from build123d import *

# Parameters (mm, degrees)
SKETCH1_R                    = 11.5
BOSS_EXTRUDE1_DEPTH          = 100
FILLET1_R                    = 8
SKETCH2_R                    = 4.1
SKETCH2_R_2                  = 6
CUT_EXTRUDE1_DEPTH           = 10
BOSS_EXTRUDE2_START          = 20
SKETCH3_R                    = 4.1
SKETCH3_R_2                  = 6
BOSS_EXTRUDE2_DEPTH          = 20
FILLET2_R                    = 3
CUT_EXTRUDE_THIN1_DEPTH      = 184.360351078
CUT_EXTRUDE_THIN1_DEPTH_BACK = 20
CUT_EXTRUDE_THIN2_DEPTH      = 164.298096582
CUT_EXTRUDE_THIN2_DEPTH_BACK = 20
FILLET3_R                    = 3
CUT_EXTRUDE2_DEPTH           = 161.944923335
CUT_EXTRUDE2_DEPTH_BACK      = 161.944923335
SKETCH6_R                    = 2.25
CUT_EXTRUDE3_DEPTH           = 3


with BuildPart() as part:
    # Sketch1 → Boss-Extrude1 (new body)
    with BuildSketch(Plane(origin=(0, 0, 0), x_dir=(1, 0, 0), z_dir=(0, 1, 0))):
        with BuildLine():
            Line((137.460581558, -14.5), (119.460581558, -14.5))
            Line((119.460581558, -14.5), (119.460581558, 11.5))
            Line((119.460581558, 11.5), (-24.539418442, 11.5))
            Line((-24.539418442, 11.5), (-24.539418442, -14.5))
            Line((-24.539418442, -14.5), (-42.539418442, -14.5))
            ThreePointArc((-42.539418442, -14.5), (-57.039418442, 0), (-42.539418442, 14.5))
            Line((-42.539418442, 14.5), (137.460581558, 14.5))
            ThreePointArc((137.460581558, 14.5), (151.960581558, 0), (137.460581558, -14.5))
        make_face()
        with Locations(Location((-42.539418442, 0, 0), (0, 0, 270))):
            Circle(SKETCH1_R, mode=Mode.SUBTRACT)
        with Locations(Location((137.460581558, 0, 0), (0, 0, 270))):
            Circle(SKETCH1_R, mode=Mode.SUBTRACT)
    extrude(amount=BOSS_EXTRUDE1_DEPTH)

    # Fillet1
    fillet1_edges = [part.edges().sort_by_distance(p)[0] for p in [
        (119.460581558, 50, 14.5),
        (119.460581558, 50, -11.5),
        (-24.539418442, 50, -11.5),
        (-24.539418442, 50, 14.5),
    ]]
    fillet(fillet1_edges, radius=FILLET1_R)

    # Sketch2 → Cut-Extrude1 (cut)
    with BuildSketch(Plane.XY.offset(-11.5)):
        with Locations((12.460581558, 50)):
            Circle(SKETCH2_R)
        with Locations((82.460581558, 50)):
            Circle(SKETCH2_R)
        with Locations((47.460581558, 50)):
            Circle(SKETCH2_R_2)
    extrude(amount=-CUT_EXTRUDE1_DEPTH, mode=Mode.SUBTRACT)

    # Sketch3 → Boss-Extrude2 (add)
    with BuildSketch(Plane.XY.offset(-11.5).offset(BOSS_EXTRUDE2_START)):
        Polygon((12.460581558, 58), (82.460581558, 58), (124.149440998, 58), (124.149440998, 42), (82.460581558, 42), (12.460581558, 42), (-28.8662965, 42), (-28.8662965, 58), (-16.539418442, 58), align=None)
        with Locations((12.460581558, 50)):
            Circle(SKETCH3_R, mode=Mode.SUBTRACT)
        with Locations((82.460581558, 50)):
            Circle(SKETCH3_R, mode=Mode.SUBTRACT)
        with Locations((47.460581558, 50)):
            Circle(SKETCH3_R_2, mode=Mode.SUBTRACT)
    extrude(amount=-BOSS_EXTRUDE2_DEPTH)

    # Fillet2
    fillet2_edges = [part.edges().sort_by_distance(p)[0] for p in [
        (-24.603180872, 58, 7.50803434),
        (-24.603180872, 42, 7.50803434),
        (47.460581558, 42, -11.5),
        (117.117435807, 42, -9.156854249),
        (119.460581558, 42, 1.5),
        (-24.539418442, 42, 1.5),
        (-22.196272692, 42, -9.156854249),
        (119.524343988, 42, 7.50803434),
        (119.460581558, 58, 1.5),
        (117.117435807, 58, -9.156854249),
        (47.460581558, 58, -11.5),
        (-22.196272692, 58, -9.156854249),
        (-24.539418442, 58, 1.5),
        (119.524343988, 58, 7.50803434),
    ]]
    fillet(fillet2_edges, radius=FILLET2_R)

    # Sketch4 → Cut-Extrude-Thin1 (cut, two sides: drawn at the far end of the back side and taken through both)
    with BuildSketch(Plane.XY.offset(8.5).offset(-CUT_EXTRUDE_THIN1_DEPTH_BACK)):
        Polygon((92.460581558, 51), (47.460581558, 51), (2.460581558, 51), (2.460581558, 49), (47.460581558, 49), (92.460581558, 49), align=None)
    extrude(amount=CUT_EXTRUDE_THIN1_DEPTH + CUT_EXTRUDE_THIN1_DEPTH_BACK, mode=Mode.SUBTRACT)

    # Sketch5 → Cut-Extrude-Thin2 (cut, two sides: drawn at the far end of the back side and taken through both)
    with BuildSketch(Plane(origin=(0, 42, 0), x_dir=(-1, 0, 0), z_dir=(0, -1, 0)).offset(-CUT_EXTRUDE_THIN2_DEPTH_BACK)):
        Polygon((-2.460581558, 8.5), (-47.460581558, 8.5), (-92.460581558, 8.5), (-92.460581558, 11.5), (-47.460581558, 11.5), (-2.460581558, 11.5), align=None)
    extrude(amount=CUT_EXTRUDE_THIN2_DEPTH + CUT_EXTRUDE_THIN2_DEPTH_BACK, mode=Mode.SUBTRACT)

    # Fillet3
    fillet3_edges = [part.edges().sort_by_distance(p)[0] for p in [
        (2.460581558, 50, -11.5),
        (92.460581558, 50, -11.5),
    ]]
    fillet(fillet3_edges, radius=FILLET3_R - 0.0001)  # a hair under: the kernel refuses the full size

    # Sketch6 → Cut-Extrude2 (cut, two sides: drawn at the far end of the back side and taken through both)
    with BuildSketch(Plane(origin=(0, 49, 0), x_dir=(1, 0, 0), z_dir=(0, 1, 0)).offset(-CUT_EXTRUDE2_DEPTH_BACK)):
        with Locations(Location((28.990631201, 0, 0), (0, 0, 270))):
            Circle(SKETCH6_R)
        with Locations(Location((65.930531914, 0, 0), (0, 0, 270))):
            Circle(SKETCH6_R)
    extrude(amount=CUT_EXTRUDE2_DEPTH + CUT_EXTRUDE2_DEPTH_BACK, mode=Mode.SUBTRACT)

    # Sketch7 → Cut-Extrude3 (cut)
    with BuildSketch(Plane(origin=(0, 58, 0), x_dir=(1, 0, 0), z_dir=(0, 1, 0))):
        Polygon((33.263023193, 0), (31.126827197, 3.7), (26.854435205, 3.7), (24.718239209, 0), (26.854435205, -3.7), (31.126827197, -3.7), align=None)
        Polygon((70.202923906, 0), (68.06672791, 3.7), (63.794335918, 3.7), (61.658139922, 0), (63.794335918, -3.7), (68.06672791, -3.7), align=None)
    extrude(amount=-CUT_EXTRUDE3_DEPTH, mode=Mode.SUBTRACT)


solid = part.part
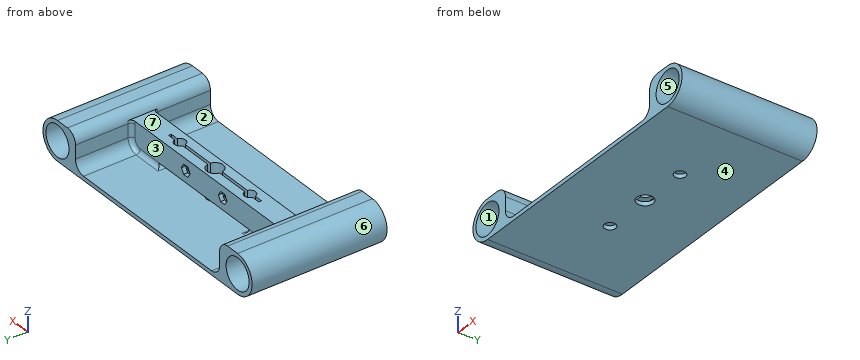
For this review, take the finished solid that the model builds, in its own axes (mm). Face numbers are marked on the shaded views. A direction names the side the tool comes from. Round coordinates to 2 decimals unless told otherwise and drop trailing zeros. Write each loop counter-clockwise with the first axis right and the second up, starting at its lowest first coordinate (ties: lowest second). Pieces come first, ordered by that corner, then holes. Notation, with made-up numbers: (-32.75, 1.5) - (-17.75, 1.5) arc R24 ccw to (-17.75, 28.5) - close; hole circle Ø9 at (1, 26.25). An arc over 180 degrees is marked (long way). Use a Markdown table: item, result.
Q1. The part is to be moulded in two halves that separate along X. For the marked faces 4, 5, 6 and 7, say which applies: pulls with the +X half, pulls with the -X half, needs draft (parallel to the pull), parting line crosses it, or undercut.
Derived:
| item | result |
|---|---|
| face 4 | needs draft |
| face 5 | undercut |
| face 6 | pulls with the -X half |
| face 7 | undercut |
Q2. We need section A-A (y = 15). Give the boundary of the cut face in (x, z), plus the area to 3 significant figures.
Derived:
| item | result |
|---|---|
| outline | (-42.54, -14.5) - (137.46, -14.5) arc R14.5 ccw to (137.46, 14.5) - (127.46, 14.5) arc R8 ccw to (119.46, 6.5) - (119.46, -3.5) arc R8 cw to (111.46, -11.5) - (-16.54, -11.5) arc R8 cw to (-24.54, -3.5) - (-24.54, 6.5) arc R8 ccw to (-32.54, 14.5) - (-42.54, 14.5) arc R14.5 ccw to start; hole circle Ø23 at (-42.54, 0); hole circle Ø23 at (137.46, 0) |
| area | 1,310 mm2 |
Q3. We need section B-B (x = 135). Give the boundary of the cut face in (y, z), plus the area to 3 significant figures.
Derived:
| item | result |
|---|---|
| outline | (0, -14.5) - (100, -14.5) - (100, -11.23) - (0, -11.23) - close; (0, 11.23) - (100, 11.23) - (100, 14.5) - (0, 14.5) - close |
| area | 653 mm2 |
Q4. Clearance check with flat-ended pins moving along their axes: pin 1 (3 mm diameter, centred on x = 6.5, z = 0, fed in from -Y); pin 2 (1.5 mm diameter, centred on x = 107.5, z = -10, fed in from +Y); pin 3 (8 mm diameter, centred on x = 20, z = -5, fed in from +Y); pin 4 (8 mm diameter, centred on y = 24.5, z = 2, fed in from +X). State where each tip first meets the part, or that it passes through.
Derived:
| item | result |
|---|---|
| pin 1 | stops at y = 42 |
| pin 2 | stops at y = 59.02 |
| pin 3 | stops at y = 58 |
| pin 4 | stops at x = 151.96 |
Q5. Machinability: for the marked faces 1, 2 and 3, which of the approach directions +Z, -Z, +X, -X, +Y, -Y give a long, thin tool a straight path to every point of the face, cutting with its end or side? Answer none if there is none.
Derived:
| item | result |
|---|---|
| face 1 | +Y, -Y |
| face 2 | +Z, -Y |
| face 3 | +Z, +Y |
Q6. Wall thickness on line 1 along Y through (x, z) = (74, -5.25); line 2 along X through (y, z) = (57.5, -7); line 3 along Z through (x, y) = (-43, 41.5): over which ranges is each line inside the solid? List them lowest first.
Derived:
| item | result |
|---|---|
| line 1 | y = 42 to 49, 51 to 58 |
| line 2 | x = -55.24 to -51.66, -33.42 to 128.34, 146.58 to 150.16 |
| line 3 | z = -14.49 to -11.49, 11.49 to 14.49 |
